Build history of the part. All positions in model axes, mm. A direction names the side the tool comes from. Round coordinates to 2 decimals unless told otherwise and drop trailing zeros. Write each loop counter-clockwise with the first axis right and the second up, starting at its lowest first coordinate (ties: lowest second). Pieces come first, ordered by that corner, then holes. Notation, with made-up numbers: (-2.75, 5) -> (45.25, 5) arc R23 cw to (45.25, 43) -> close; hole circle Ø1 at (-39, 23.25). An arc over 180 degrees is marked (long way). Answer in a Markdown table with one row per item. Add a question column.
from build123d import *


with BuildPart() as part:
    # Croquis1 → Revolución1 (revolve)
    with BuildSketch(Plane.XY, mode=Mode.PRIVATE) as revoluci_n1_sk:
        with BuildLine():
            Line((-8.065, 0), (-13.45, 0))
            ThreePointArc((-13.45, 0), (-13.646270241, -0.028078879), (-13.826794629, -0.110062878))
            Line((-13.826794629, -0.110062878), (-20.7, -4.5))
            Line((-20.7, -4.5), (-27, -4.5))
            Line((-27, -4.5), (-27, -3))
            Line((-27, -3), (-27.7, -3))
            Line((-27.7, -3), (-27.7, -4.5))
            ThreePointArc((-27.7, -4.5), (-27.494974747, -4.994974747), (-27, -5.2))
            Line((-27, -5.2), (-20.7, -5.2))
            ThreePointArc((-20.7, -5.2), (-20.503729759, -5.171921121), (-20.323205371, -5.089937122))
            Line((-20.323205371, -5.089937122), (-13.45, -0.7))
            Line((-13.45, -0.7), (-8.065, -0.7))
            Line((-8.065, -0.7), (-8.065, 0))
        make_face()
    revolve(revoluci_n1_sk.sketch.rotate(Axis((0, 0, 0), (0, 1, 0)), 270), axis=Axis((0, 0, 0), (0, 1, 0)))


solid = part.part
(1) Saw through at B-B (x = 0). List the corners of the cut face in (y, z) (3 decimals).
(2) Probe line 1 along Z through (x, y) = (-11, -4.25); line 2 along Z through (x, y) = (2, -4.05); line 3 along Y through (x, z) = (16.5, 14). List the from-to ranges inside material, lowest first.
(3) Drop flat-ended pins along their axis: P1, Ø1, axis at x = -2.5, y = -0.5, coming from the +Z side; P2, Ø18.5, axis at x = 0, z = 0, coming from the -Y side; P3, Ø1.5, axis at y = -1.5, z = -9, coming from the -X side; P4, Ø5, axis at x = -19.5, z = -5.5, coming from the -Y side. Give the stop position or say it passes through.
(4) Mould opens along X. For faces 1 (the face through (27.041, -3.76, 6.005)), 2 (the face through (6, -3, 26.5)), 3 (the face through (-2.4, -0.3, -7.7)) say: pulls with the +X half, pulls with the -X half, needs draft (parallel to the pull), parting line crosses it, or undercut.
(5) Which spindle directions (+Z, -Z, +X, -X, +Y, -Y) get a long thin tool onto all of the face, cutting with end or side? Do faces 4 (the face through (20, -5.2, 6)), 5 (the face through (6, -0.7, -6)), 6 (the face through (20, -4.5, -6)). Say none if no direction does.
(6) Saw through at A-A (z = 0). List the corners of the cut face in (x, y) (3 decimals).
Answer sheet:
| question | item | result |
|---|---|---|
| 1 | outline | (-5.2, -27) arc R0.7 ccw to (-4.5, -27.7) -> (-3, -27.7) -> (-3, -27) -> (-4.5, -27) -> (-4.5, -20.7) -> (-0.11, -13.827) arc R0.7 ccw to (0, -13.45) -> (0, -8.065) -> (-0.7, -8.065) -> (-0.7, -13.45) -> (-5.09, -20.323) arc R0.7 ccw to (-5.2, -20.7) -> close; (-5.2, 20.7) arc R0.7 ccw to (-5.09, 20.323) -> (-0.7, 13.45) -> (-0.7, 8.065) -> (0, 8.065) -> (0, 13.45) arc R0.7 ccw to (-0.11, 13.827) -> (-4.5, 20.7) -> (-4.5, 27) -> (-3, 27) -> (-3, 27.7) -> (-4.5, 27.7) arc R0.7 ccw to (-5.2, 27) -> close |
| 2 | line 1 | z = -25.42 to -24.66, -17.07 to -15.5, 15.5 to 17.07, 24.66 to 25.42 |
| 2 | line 2 | z = -27.63 to -26.93, -19.9 to -18.59, 18.59 to 19.9, 26.93 to 27.63 |
| 2 | line 3 | y = -5.2 to -4.5 |
| 3 | P1 | stops at z = 15.02 |
| 3 | P2 | stops at y = -0.7 |
| 3 | P3 | stops at x = -14.7 |
| 3 | P4 | stops at y = -5.2 |
| 4 | face 1 | parting line crosses it |
| 4 | face 2 | needs draft |
| 4 | face 3 | undercut |
| 5 | face 4 | +Z, -Z, +X, -X, -Y |
| 5 | face 5 | -Y |
| 5 | face 6 | +Y |
| 6 | outline | (-27.7, -4.5) arc R0.7 ccw to (-27, -5.2) -> (-20.7, -5.2) arc R0.7 ccw to (-20.323, -5.09) -> (-13.45, -0.7) -> (-8.065, -0.7) -> (-8.065, 0) -> (-13.45, 0) arc R0.7 ccw to (-13.827, -0.11) -> (-20.7, -4.5) -> (-27, -4.5) -> (-27, -3) -> (-27.7, -3) -> close; (8.065, -0.7) -> (13.45, -0.7) -> (20.323, -5.09) arc R0.7 ccw to (20.7, -5.2) -> (27, -5.2) arc R0.7 ccw to (27.7, -4.5) -> (27.7, -3) -> (27, -3) -> (27, -4.5) -> (20.7, -4.5) -> (13.827, -0.11) arc R0.7 ccw to (13.45, 0) -> (8.065, 0) -> close |
